Autodesk Inventor part; units mm, degrees
ref_plane "YZ Plane" through (0, 0, 0) normal (1, 0, 0) x (0, 1, 0)
ref_plane "XZ Plane" through (0, 0, 0) normal (0, 1, 0) x (-1, 0, 0)
ref_plane "XY Plane" through (0, 0, 0) normal (0, 0, 1) x (1, 0, 0)
ref_plane "Work Plane1" through (0, 0, 0) normal (0, 0, 1) x (1, 0, 0)
sketch "Sketch1" plane through (0, 0, 0) normal (0, 0, 1) x (1, 0, 0)
  line L0 (14.1799, -15.6518) -> (35.3799, -15.6518)
  line L1 (35.3799, -15.6518) -> (35.3799, -31.6518)
  line L2 (35.3799, -31.6518) -> (14.1799, -31.6518)
  line L3 (14.1799, -31.6518) -> (14.1799, -15.6518)
  point P0 (0, 0)
  dimension "d0" = 21.2
  dimension "d2" = 16
extrude "Extrusion1" add sketch "Sketch1" along normal blind 13.4
sketch "Sketch2" plane through (35.3799, -31.6518, 0) normal (1, 0, 0) x (0, 0, -1)
  line L0 (0, 16) -> (0, 0)
  line L1 (0, 16) -> (-13.4, 16)
  line L2 (-13.4, 0) -> (-13.4, 16)
  line L3 (0, 0) -> (-13.4, 0)
  line L4 (-10.9, 2) -> (-4.3, 2)
  line L5 (-4.3, 2) -> (-4.3, 5)
  line L6 (-4.3, 5) -> (-2.5, 5)
  line L7 (-2.5, 5) -> (-2.5, 6)
  line L8 (-2.5, 6) -> (-1, 6)
  line L9 (-1, 6) -> (-1, 10)
  line L10 (-1, 10) -> (-2.5, 10)
  line L11 (-2.5, 10) -> (-2.5, 11)
  line L12 (-2.5, 11) -> (-4.3, 11)
  line L13 (-4.3, 11) -> (-4.3, 14)
  line L14 (-4.3, 14) -> (-10.9, 14)
  line L15 (-10.9, 14) -> (-10.9, 2)
  point P0 (0, 31.6518)
  dimension "d5" = 2
  dimension "d6" = 2
  dimension "d7" = 2.5
  dimension "d8" = 5
  dimension "d9" = 6
  dimension "d10" = 1
  dimension "d11" = 2.5
  dimension "d12" = 4.3
extrude "Extrusion2" cut sketch "Sketch2" against normal blind 11.5 contours L15 L14 L13 L12 L11 L10 L9 L8 L7 L6 L5 L4
sketch "Sketch3" plane through (35.3799, -31.6518, 0) normal (1, 0, 0) x (0, 0, -1)
  line L0 (-4.3, 5) -> (-4.3, 2)
  line L1 (-4.3, 2) -> (-10.9, 2)
  line L2 (-10.9, 14) -> (-4.3, 14)
  line L3 (-4.3, 14) -> (-4.3, 11)
  line L4 (-4.3, 11) -> (-2.5, 11)
  line L5 (-2.5, 5) -> (-4.3, 5)
  line L6 (-4.1, 4.8) -> (-2.5, 4.8)
  line L7 (-2.5, 4.8) -> (-2.5, 2)
  line L8 (-2.5, 2) -> (-4.1, 2)
  line L9 (-4.1, 2) -> (-4.1, 4.8)
  line L10 (-4.1, 11.2) -> (-2.5, 11.2)
  line L11 (-2.5, 11.2) -> (-2.5, 14)
  line L12 (-2.5, 14) -> (-4.1, 14)
  line L13 (-4.1, 14) -> (-4.1, 11.2)
  point P0 (0, 31.6518)
  dimension "d15" = 0.2
  dimension "d16" = 0.2
  dimension "d17" = 0.2
  dimension "d18" = 0.2
extrude "Extrusion3" cut sketch "Sketch3" against normal blind 0.2
properties part number "nanopc_t4_rj45"
Part model, mm, in its own coordinate system. A direction names the side the tool comes from. Round coordinates to 2 decimals unless told otherwise and drop trailing zeros. Loops run counter-clockwise (first coordinate to the right, second up) from the corner with the lowest first, then second, coordinate; pieces in that order, holes last. Notation, with made-up numbers: (44, -18) -> (83, -18) arc R18 ccw to (83, -11) -> close; hole circle Ø2 at (-28.5, 13.25). An arc over 180 degrees is marked (long way). Use a Markdown table: item, result.
1) Cut at D-D, the plane z = 3.75. List the corners of the cut face in (x, y), and give its area (3 significant figures).
The answers:
| item | result |
|---|---|
| outline | (14.18, -31.65) -> (35.38, -31.65) -> (35.38, -29.65) -> (35.18, -29.65) -> (35.18, -26.85) -> (35.38, -26.85) -> (35.38, -26.65) -> (23.88, -26.65) -> (23.88, -20.65) -> (35.38, -20.65) -> (35.38, -20.45) -> (35.18, -20.45) -> (35.18, -17.65) -> (35.38, -17.65) -> (35.38, -15.65) -> (14.18, -15.65) -> close |
| area | 269 mm2 |
2) Drop a flat-ended pin along its axis: pin 1 Ø2 at (y, z) = (-20, 9.5) entering from +X. Give the stop position or say it passes through.
The answers:
| item | result |
|---|---|
| pin 1 | stops at x = 23.88 |
3) Tool access for faces 4 (the flat face through (30, -21, 2.5)), 5 (the flat face through (25, -31.652, 7)): list every direction of +Z, -Z, +X, -X, +Y, -Y with a clear straight run to the whole face (end or side of a thin tool).
The answers:
| item | result |
|---|---|
| face 4 | +X |
| face 5 | +Z, -Z, +X, -X, -Y |
4) Cut at A-A, the plane z = 2. List the corners of the cut face in (x, y), and give its area (3 significant figures).
The answers:
| item | result |
|---|---|
| outline | (14.18, -31.65) -> (35.38, -31.65) -> (35.38, -25.65) -> (23.88, -25.65) -> (23.88, -21.65) -> (35.38, -21.65) -> (35.38, -15.65) -> (14.18, -15.65) -> close |
| area | 293 mm2 |
5) Pull direction Y, two halves, no side cores. Call faces 1 (the flat face through (30, -26, 2.5)), 2 (the flat face through (25, -24, 13.4)), 3 (the flat face through (25, -15.652, 7)): pulls with the +Y half, pulls with the -Y half, needs draft (parallel to the pull), parting line crosses it, or undercut.
The answers:
| item | result |
|---|---|
| face 1 | undercut |
| face 2 | needs draft |
| face 3 | pulls with the +Y half |
6) Cut at C-C, the plane y = -22.5. List the corners of the cut face in (x, z).
The answers:
| item | result |
|---|---|
| outline | (14.18, 0) -> (35.38, 0) -> (35.38, 1) -> (23.88, 1) -> (23.88, 10.9) -> (35.38, 10.9) -> (35.38, 13.4) -> (14.18, 13.4) -> close |
7) Cut at B-B, the plane x = 26. List the corners of the cut face in (y, z), and give its area (3 significant figures).
The answers:
| item | result |
|---|---|
| outline | (-31.65, 0) -> (-15.65, 0) -> (-15.65, 13.4) -> (-31.65, 13.4) -> close; hole (-29.65, 4.3) -> (-26.65, 4.3) -> (-26.65, 2.5) -> (-25.65, 2.5) -> (-25.65, 1) -> (-21.65, 1) -> (-21.65, 2.5) -> (-20.65, 2.5) -> (-20.65, 4.3) -> (-17.65, 4.3) -> (-17.65, 10.9) -> (-29.65, 10.9) -> close |
| area | 118 mm2 |
8) Probe line 1 (Z direction, x = 24.75, y = -27.5); line 2 (Z direction, x = 26.25, y = -25); line 3 (Y direction, x = 33.5, z = 7.25). List the from-to ranges inside material, lowest first. Write a range as [from, to].
The answers:
| item | result |
|---|---|
| line 1 | z = [0, 4.3], [10.9, 13.4] |
| line 2 | z = [0, 1], [10.9, 13.4] |
| line 3 | y = [-31.65, -29.65], [-17.65, -15.65] |
